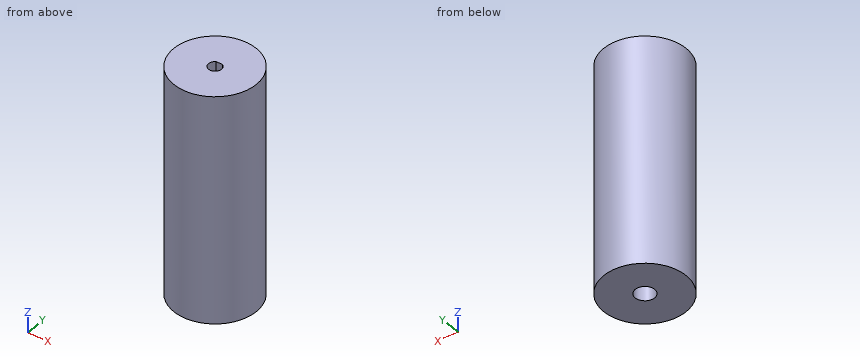
```python
from build123d import *

# Parameters (mm, degrees)
SKETCH1_R           = 12.7
BOSS_EXTRUDE1_DEPTH = 69.85
CUT_EXTRUDE1_DEPTH  = 10
SKETCH3_R           = 2.999994
CUT_EXTRUDE2_DEPTH  = 34.925


with BuildPart() as part:
    # Sketch1 → Boss-Extrude1 (new body)
    with BuildSketch(Plane.XY):
        Circle(SKETCH1_R)
    extrude(amount=BOSS_EXTRUDE1_DEPTH)

    # Sketch2 → Cut-Extrude1 (cut)
    with BuildSketch(Plane.XY.offset(69.85)):
        with BuildLine():
            Line((-0.968245837, 1.75), (0.968245837, 1.75))
            ThreePointArc((0.968245837, 1.75), (0, -2), (-0.968245837, 1.75))
        make_face()
    extrude(amount=-CUT_EXTRUDE1_DEPTH, mode=Mode.SUBTRACT)

    # Sketch3 → Cut-Extrude2 (cut)
    with BuildSketch(Plane(origin=(0, 0, 0), x_dir=(-1, 0, 0), z_dir=(0, 0, -1))):
        Circle(SKETCH3_R)
    extrude(amount=-CUT_EXTRUDE2_DEPTH, mode=Mode.SUBTRACT)


solid = part.part
```
The model under review builds one solid part; all positions refer to its coordinate system, in mm. Give positions to 0.01 mm unless a question says otherwise; leave off trailing zeros. Write each loop counter-clockwise with the first axis right and the second up, starting at its lowest first coordinate (ties: lowest second). Pieces come first, ordered by that corner, then holes. Notation, with made-up numbers: (26.5, -17) -> (61.5, -17) arc R22 ccw to (61.5, 7) -> close; hole circle Ø6 at (88, 87.25). An arc over 180 degrees is marked (long way). Answer in a Markdown table with one row per item.
1) Add section D-D on z = 21. State the section outline as (x, y) points.
Worked answers:
| item | result |
|---|---|
| outline | circle Ø25.4 at (0, 0); hole circle Ø6 at (0, 0) |
2) Add section B-B on x = 0. State the section outline as (y, z) points (3 decimals).
Worked answers:
| item | result |
|---|---|
| outline | (-12.7, 0) -> (-3, 0) -> (-3, 34.925) -> (3, 34.925) -> (3, 0) -> (12.7, 0) -> (12.7, 69.85) -> (1.75, 69.85) -> (1.75, 59.85) -> (-2, 59.85) -> (-2, 69.85) -> (-12.7, 69.85) -> close |
3) Add section A-A on y = 0. State the section outline as (x, z) points (3 decimals).
Worked answers:
| item | result |
|---|---|
| outline | (-12.7, 0) -> (-3, 0) -> (-3, 34.925) -> (3, 34.925) -> (3, 0) -> (12.7, 0) -> (12.7, 69.85) -> (2, 69.85) -> (2, 59.85) -> (-2, 59.85) -> (-2, 69.85) -> (-12.7, 69.85) -> close |
4) Add section C-C on z = 41. State the section outline as (x, y) points.
Worked answers:
| item | result |
|---|---|
| outline | circle Ø25.4 at (0, 0) |
5) Clearance check with flat-ended pins moving along their axes: P1, Ø5, axis at x = 0, y = 0, coming from the -Z side (3 decimals); P2, Ø1.5, axis at x = 8, z = 38.5, coming from the +Y side; P3, Ø5, axis at y = 8, z = 54, coming from the +X side. State where each tip first meets the part, or that it passes through.
Worked answers:
| item | result |
|---|---|
| P1 | z = 34.925 |
| P2 | y = 10.43 |
| P3 | x = 11.45 |
6) For L1, parallel to Y at x = 0, z = 9; L2, parallel to Z at x = -2.75, y = -0.25 (3 decimals); L3, parallel to Y at x = -10.5, z = 26, list the stretches that pass through material, from the lowest coordinate up. Write a range as [from, to].
Worked answers:
| item | result |
|---|---|
| L1 | [-12.7, -3], [3, 12.7] |
| L2 | [34.925, 69.85] |
| L3 | [-7.14, 7.14] |
